Print and shaded views of the part. All mm, measured from the part's lowest x, y and z. Give positions to 0.01 mm unless a question says otherwise; leave off trailing zeros. Order: outer loops, then holes, each group sorted by start corner. A loop starts at its lowest first (then second) coordinate and runs counter-clockwise, first axis right, second up. Notation, with made-up numbers: (73.25, -22.75) -> (122.25, -22.75) arc R35 ccw to (122.25, 10.25) -> close; hole circle Ø10 at (-20.75, -23). An arc over 180 degrees is marked (long way). One line per question, with ' | ' between items. Start each with the question number.
(1) Cut at C-C (x = 62.5). Give the cut face in (y, z) (1 decimal).
(2) Drill centre lines: L1, parallel to X at y = 2.1, z = 26.5; L2, parallel to X at y = 2.6, z = 28; L3, parallel to Z at x = 34, y = 1.35 (3 decimals). Where is each one in solid material? Low to high. Write a range as from..to.
(3) Cut at A-A (x = 35.5). Give the cut face in (y, z) (3 decimals), then the cut area to 3 significant figures.
(4) Cut at B-B (y = 2.45). Give the number of separate pieces and of enclosed holes in the cut face, then the cut area to 3 significant figures.
(5) Pin check, flat tip, straight feed: pin 1 Ø1 at (x, y) = (3, 1) entering from +Z. Stop position of the tip, or through.
(6) Cut at D-D (x = 9). Give the cut face in (y, z) (3 decimals), then the cut area to 3 significant figures.
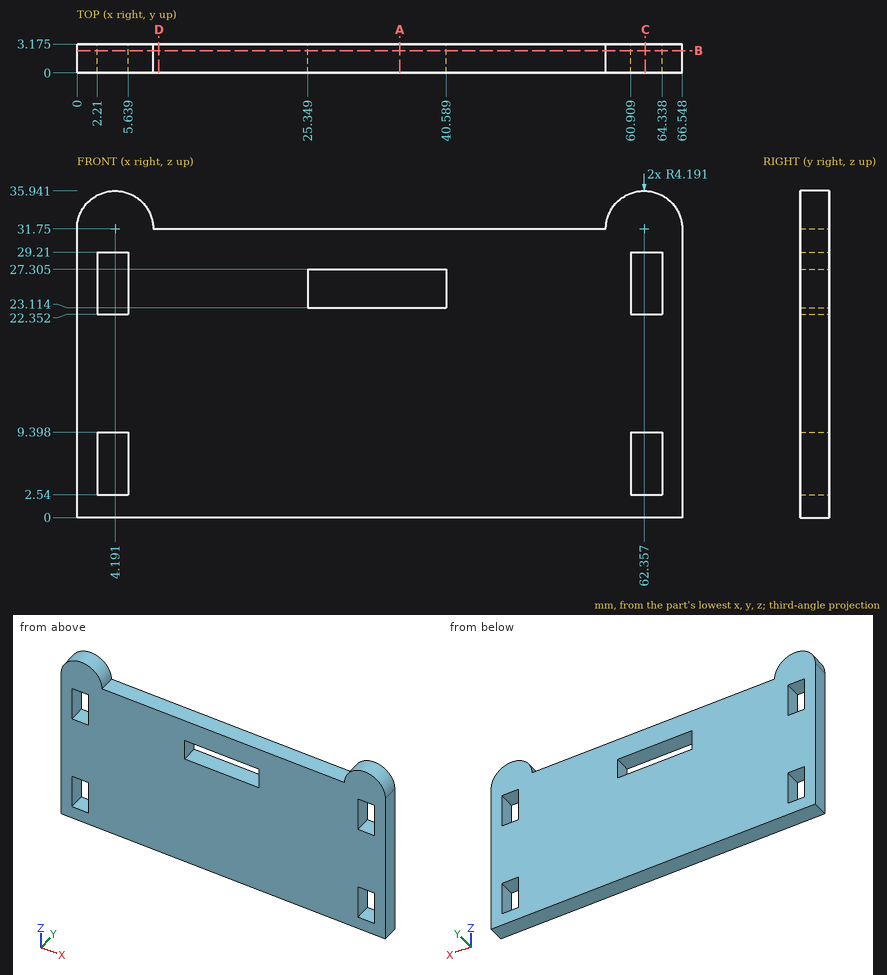
Result set:
1) outline: (0, 0) -> (3.2, 0) -> (3.2, 2.5) -> (0, 2.5) -> close; (0, 9.4) -> (3.2, 9.4) -> (3.2, 22.4) -> (0, 22.4) -> close; (0, 29.2) -> (3.2, 29.2) -> (3.2, 35.9) -> (0, 35.9) -> close
2) L1: x = 0..2.21, 5.64..25.35, 40.59..60.91, 64.34..66.55 | L2: x = 0..2.21, 5.64..60.91, 64.34..66.55 | L3: z = 0..23.114, 27.305..31.75
3) outline: (0, 0) -> (3.175, 0) -> (3.175, 23.114) -> (0, 23.114) -> close; (0, 27.305) -> (3.175, 27.305) -> (3.175, 31.75) -> (0, 31.75) -> close | area: 87.5 mm2
4) separate pieces: 1 | enclosed holes: 5 | area: 2,010 mm2
5) pin 1: stops at z = 35.88
6) outline: (0, 0) -> (3.175, 0) -> (3.175, 31.75) -> (0, 31.75) -> close | area: 101 mm2
